The listing builds one solid part. Answer for the finished solid, in the listing's coordinates (mm). Face numbers are marked on the shaded views. Round coordinates to 2 decimals unless told otherwise and drop trailing zeros. Order: outer loops, then holes, each group sorted by start corner. A loop starts at its lowest first (then second) coordinate and runs counter-clockwise, first axis right, second up. Notation, with made-up numbers: M 56,84 L 60,84 A27 ccw 60,123 Z; hole C 3,63.5 d2. An arc over 180 degrees is marked long. Put each result on its own line as item: value. Start each with the question number.
1. The part is cut by section C-C (y = 0). Give the vertices of the cut face in (x, z), then the cut area to 3 significant figures.
2. Consider line 1 (X direction, y = 1.25, z = 1); line 2 (Y direction, x = 0, z = 1.3); line 3 (X direction, y = 2, z = 4.05). Determine where each line is inside the solid, lowest interval first.
3. This flat-tipped pin is pushed along its axis until it touches: pin 1 Ø1.5 at (x, y) = (2, -3) entering from +Z. Where does it stop, or does it pass through?
4. The mould has two halves that part along Y. Classify the marked faces 1, 2, 3 and 4: +Y half, -Y half, draft (parallel to the pull), parting line (faces both ways), or undercut.
5. The part is cut by section A-A (z = 0.3). Give the vertices of the cut face in (x, y).
6. The part is cut by section B-B (x = 0). Give the vertices of the cut face in (y, z).
7. The part is cut by section D-D (z = 2.05). Give the vertices of the cut face in (x, y).
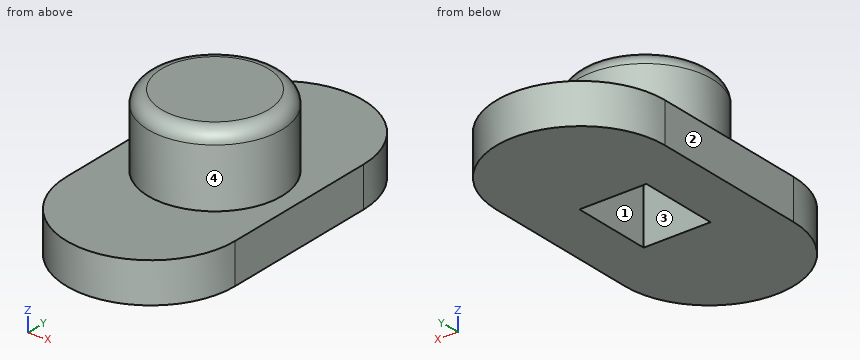
from build123d import *

# Parameters (mm, degrees)
F0_R     = 2.5
F0_W     = 2.5
F0_H     = 3
F1_DEPTH = 1.5
F2_DEPTH = 4.2
F3_DEPTH = 2.5
F4_R     = 0.5


with BuildPart() as f1:
    # F0 (on Top) → F1 (new body)
    with BuildSketch(Plane.XY):
        with BuildLine():
            Line((-3.15, 3), (-3.15, -3))
            ThreePointArc((-3.15, -3), (0, -6.15), (3.15, -3))
            Line((3.15, -3), (3.15, 3))
            ThreePointArc((3.15, 3), (0, 6.15), (-3.15, 3))
        make_face()
        Circle(F0_R, mode=Mode.SUBTRACT)
        Circle(F0_R)
        Rectangle(F0_W, F0_H, mode=Mode.SUBTRACT)
        Rectangle(F0_W, F0_H)
    extrude(amount=F1_DEPTH)

    # F0 (on Top) → F2 (join)
    with BuildSketch(Plane.XY):
        Circle(F0_R)
        Rectangle(F0_W, F0_H, mode=Mode.SUBTRACT)
        Rectangle(F0_W, F0_H)
    extrude(amount=F2_DEPTH)

    # F0 (on Top) → F3 (cut)
    with BuildSketch(Plane.XY):
        Rectangle(F0_W, F0_H)
    extrude(amount=F3_DEPTH, mode=Mode.SUBTRACT)

    # F4
    f4_edges = [f1.edges().sort_by_distance(p)[0] for p in [
        (-2.5, 0, 4.2),
    ]]
    fillet(f4_edges, radius=F4_R)


solid = f1.part
Resolved:
1. outline: M -3.15,0 L -1.25,0 L -1.25,2.5 L 1.25,2.5 L 1.25,0 L 3.15,0 L 3.15,1.5 L 2.5,1.5 L 2.5,3.7 A0.5 ccw 2,4.2 L -2,4.2 A0.5 ccw -2.5,3.7 L -2.5,1.5 L -3.15,1.5 Z
1. area: 16.6 mm2
2. line 1: -3.15 to -1.25, 1.25 to 3.15
2. line 2: -6.15 to -1.5, 1.5 to 6.15
2. line 3: -1.25 to 1.25
3. pin 1: z = 1.5
4. face 1: undercut
4. face 2: draft
4. face 3: undercut
4. face 4: parting line
5. outline: M -3.15,-3 A3.15 ccw 3.15,-3 L 3.15,3 A3.15 ccw -3.15,3 Z; hole M -1.25,-1.5 L 1.25,-1.5 L 1.25,1.5 L -1.25,1.5 Z
6. outline: M -6.15,0 L -1.5,0 L -1.5,2.5 L 1.5,2.5 L 1.5,0 L 6.15,0 L 6.15,1.5 L 2.5,1.5 L 2.5,3.7 A0.5 ccw 2,4.2 L -2,4.2 A0.5 ccw -2.5,3.7 L -2.5,1.5 L -6.15,1.5 Z
7. outline: C 0,0 d5; hole M -1.25,-1.5 L 1.25,-1.5 L 1.25,1.5 L -1.25,1.5 Z
